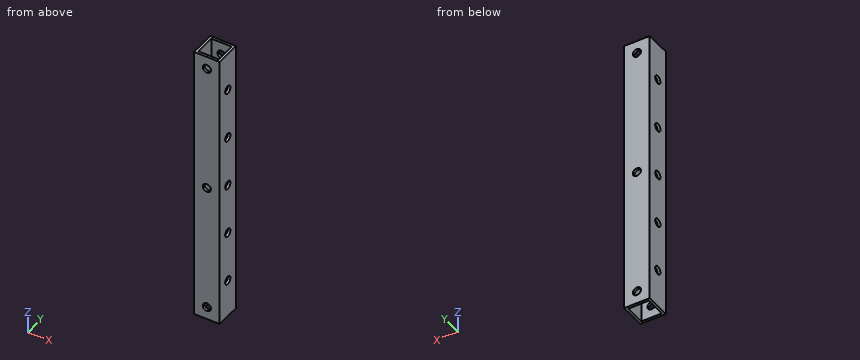
```python
from build123d import *

# Parameters (mm, degrees)
SKETCH1_W           = 10
SKETCH1_H           = 10
BOSS_EXTRUDE1_DEPTH = 55
SKETCH2_W           = 8
SKETCH2_H           = 8
CUT_EXTRUDE1_DEPTH  = 110
SKETCH4_R           = 1.6
CUT_EXTRUDE2_DEPTH  = 10
SKETCH3_R           = 1.6
CUT_EXTRUDE3_DEPTH  = 10


with BuildPart() as part:
    # Sketch1 → Boss-Extrude1 (new body)
    with BuildSketch(Plane.XY):
        with Locations((-26.52173913, 10.217391304)):
            Rectangle(SKETCH1_W, SKETCH1_H)
    boss_extrude1 = extrude(amount=BOSS_EXTRUDE1_DEPTH)

    # Sketch2 → Cut-Extrude1 (cut)
    with BuildSketch(Plane.XY.offset(55)):
        with Locations((-26.517415058, 10.213067232)):
            Rectangle(SKETCH2_W, SKETCH2_H)
    cut_extrude1 = extrude(amount=-CUT_EXTRUDE1_DEPTH, mode=Mode.SUBTRACT)

    # Sketch4 → Cut-Extrude2 (cut)
    with BuildSketch(Plane(origin=(-21.52173913, 0, 0), x_dir=(0, 0, -1), z_dir=(1, 0, 0))):
        with Locations((-15, 10.217391304)):
            Circle(SKETCH4_R)
        with Locations((-35, 10.217391304)):
            Circle(SKETCH4_R)
        with Locations((-55, 10.217391304)):
            Circle(SKETCH4_R)
    cut_extrude2 = extrude(amount=-CUT_EXTRUDE2_DEPTH, mode=Mode.SUBTRACT)

    # Sketch3 → Cut-Extrude3 (cut)
    with BuildSketch(Plane(origin=(0, 15.217391304, 0), x_dir=(1, 0, 0), z_dir=(0, 1, 0))):
        with BuildLine():
            Line((-28.12173913, -55), (-24.92173913, -55))
            ThreePointArc((-24.92173913, -55), (-26.52173913, -53.4), (-28.12173913, -55))
        make_face()
        with BuildLine():
            ThreePointArc((-28.12173913, -55), (-26.52173913, -56.6), (-24.92173913, -55))
            Line((-24.92173913, -55), (-28.12173913, -55))
        make_face()
        with Locations(Location((-26.52173913, -5, 0), (0, 0, 270))):
            Circle(SKETCH3_R)
    cut_extrude3 = extrude(amount=-CUT_EXTRUDE3_DEPTH, mode=Mode.SUBTRACT)

    # Mirror1: Boss-Extrude1, Cut-Extrude1, Cut-Extrude2, Cut-Extrude3 across plane
    add(boss_extrude1.mirror(Plane.XY.offset(55)))
    add(cut_extrude1.mirror(Plane.XY.offset(55)), mode=Mode.SUBTRACT)
    add(cut_extrude2.mirror(Plane.XY.offset(55)), mode=Mode.SUBTRACT)
    add(cut_extrude3.mirror(Plane.XY.offset(55)), mode=Mode.SUBTRACT)


solid = part.part
```
Source: CAD feature listing. Evaluate the final solid. Frame: model axes, mm. Round coordinates to 2 decimals unless told otherwise and drop trailing zeros. Loops run counter-clockwise (first coordinate to the right, second up) from the corner with the lowest first, then second, coordinate; pieces in that order, holes last. Notation, with made-up numbers: M 64,-14.75 L 109,-14.75 A29 cw 109,7.25 Z; hole C 66,48 d8. An arc over 180 degrees is marked long. Use a Markdown table: item, result. Add a question column.
1. Cut plane B-B, the plane z = 98. Output: boundary loops of the cut face in (x, y).
2. Contact query for a flat-ended pin moving along its axis: pin 1 (1 mm diameter, centred on x = -22.5, y = 10, fed in from -Z). Output: stop coordinate, or through.
3. Ray query, line 1 along X through (y, z) = (13.25, 19); line 2 along Y through (x, z) = (-30.25, 78); line 3 along Y through (x, z) = (-21.65, 35). Return the intervals inside material, ascending. Write a range as [from, to].
4. Cut plane A-A, the plane z = 5. Output: boundary loops of the cut face in (x, y), and give its area (3 significant figures).
Solution:
| question | item | result |
|---|---|---|
| 1 | outline | M -31.52,5.22 L -21.52,5.22 L -21.52,15.22 L -31.52,15.22 Z; hole M -30.52,6.21 L -22.52,6.21 L -22.52,14.21 L -30.52,14.21 Z |
| 2 | pin 1 | stops at z = 0 |
| 3 | line 1 | x = [-31.52, -30.52], [-22.52, -21.52] |
| 3 | line 2 | y = [5.22, 6.21], [14.21, 15.22] |
| 3 | line 3 | y = [5.22, 8.62], [11.82, 15.22] |
| 4 | outline | M -31.52,5.22 L -28.12,5.22 L -28.12,6.21 L -30.52,6.21 L -30.52,14.21 L -28.12,14.21 L -28.12,15.22 L -31.52,15.22 Z; M -24.92,5.22 L -21.52,5.22 L -21.52,15.22 L -24.92,15.22 L -24.92,14.21 L -22.52,14.21 L -22.52,6.21 L -24.92,6.21 Z |
| 4 | area | 29.6 mm2 |
